```python
from build123d import *

# Parameters (mm, degrees)
SKETCH3_W               = 200
SKETCH3_H               = 160
BOSS_EXTRUDE1_DEPTH     = 4
SKETCH4_R               = 2
CUT_EXTRUDE1_DEPTH      = 129.124939024
CUT_EXTRUDE3_DEPTH      = 129.124939024
CUT_EXTRUDE3_DEPTH_BACK = 129.124939024
SKETCH5_W               = 30
SKETCH5_H               = 8
SKETCH7_W               = 25
SKETCH7_H               = 74
CUT_EXTRUDE4_DEPTH      = 129.124939024
CUT_EXTRUDE6_DEPTH      = 129.124939024
CUT_EXTRUDE6_DEPTH_BACK = 4
SKETCH12_W              = 8
SKETCH12_H              = 120
CUT_EXTRUDE8_DEPTH      = 129.124939024
SKETCH14_W              = 8
SKETCH14_H              = 120
CUT_EXTRUDE9_DEPTH      = 129.124939024
SKETCH15_W              = 8
SKETCH15_H              = 40
CUT_EXTRUDE10_DEPTH     = 129.124939024
SKETCH16_W              = 35
SKETCH16_H              = 8
CUT_EXTRUDE11_DEPTH     = 129.124939024


with BuildPart() as part:
    # Sketch3 → Boss-Extrude1 (new body)
    with BuildSketch(Plane(origin=(0, 0, 0), x_dir=(1, 0, 0), z_dir=(0, 1, 0))):
        Rectangle(SKETCH3_W, SKETCH3_H)
    extrude(amount=BOSS_EXTRUDE1_DEPTH)

    # Sketch4 → Cut-Extrude1 (cut, through all)
    with BuildSketch(Plane(origin=(0, 4, 0), x_dir=(1, 0, 0), z_dir=(0, 1, 0))):
        with Locations(Location((-93, 73, 0), (0, 0, 270))):
            Circle(SKETCH4_R)
        with Locations(Location((93, 73, 0), (0, 0, 270))):
            Circle(SKETCH4_R)
        with Locations(Location((-93, -73, 0), (0, 0, 270))):
            Circle(SKETCH4_R)
        with Locations(Location((93, -73, 0), (0, 0, 270))):
            Circle(SKETCH4_R)
    extrude(amount=-CUT_EXTRUDE1_DEPTH, mode=Mode.SUBTRACT)

    # Sketch5 → Cut-Extrude3 (cut, two sides: drawn at the far end of the back side and taken through both)
    with BuildSketch(Plane(origin=(0, 4, 0), x_dir=(1, 0, 0), z_dir=(0, 1, 0)).offset(-CUT_EXTRUDE3_DEPTH_BACK)):
        with Locations((-85, 46)):
            Rectangle(SKETCH5_W, SKETCH5_H)
    extrude(amount=CUT_EXTRUDE3_DEPTH + CUT_EXTRUDE3_DEPTH_BACK, mode=Mode.SUBTRACT)

    # Sketch7 → Cut-Extrude4 (cut, through all)
    with BuildSketch(Plane(origin=(0, 4, 0), x_dir=(1, 0, 0), z_dir=(0, 1, 0))):
        with Locations((-82.5, 0)):
            Rectangle(SKETCH7_W, SKETCH7_H)
    extrude(amount=-CUT_EXTRUDE4_DEPTH, mode=Mode.SUBTRACT)

    # Sketch11 → Cut-Extrude6 (cut, two sides: drawn at the far end of the back side and taken through both)
    with BuildSketch(Plane(origin=(0, 4, 0), x_dir=(1, 0, 0), z_dir=(0, 1, 0)).offset(-CUT_EXTRUDE6_DEPTH_BACK)):
        Polygon((-587.074417675, -42), (-100, -42), (-70, -42), (-70, -50), (-100, -50), (-587.074417675, -50), (-1561.223253025, -50), (-1561.223253025, -42), align=None)
    extrude(amount=CUT_EXTRUDE6_DEPTH + CUT_EXTRUDE6_DEPTH_BACK, mode=Mode.SUBTRACT)

    # Sketch12 → Cut-Extrude8 (cut, through all)
    with BuildSketch(Plane(origin=(0, 4, 0), x_dir=(1, 0, 0), z_dir=(0, 1, 0))):
        with Locations((91, 0)):
            Rectangle(SKETCH12_W, SKETCH12_H)
    extrude(amount=-CUT_EXTRUDE8_DEPTH, mode=Mode.SUBTRACT)

    # Sketch14 → Cut-Extrude9 (cut, through all)
    with BuildSketch(Plane(origin=(0, 4, 0), x_dir=(1, 0, 0), z_dir=(0, 1, 0))):
        with Locations((38, 0)):
            Rectangle(SKETCH14_W, SKETCH14_H)
    extrude(amount=-CUT_EXTRUDE9_DEPTH, mode=Mode.SUBTRACT)

    # Sketch15 → Cut-Extrude10 (cut, through all)
    with BuildSketch(Plane(origin=(0, 4, 0), x_dir=(1, 0, 0), z_dir=(0, 1, 0))):
        with Locations((-56, -40)):
            Rectangle(SKETCH15_W, SKETCH15_H)
    extrude(amount=-CUT_EXTRUDE10_DEPTH, mode=Mode.SUBTRACT)

    # Sketch16 → Cut-Extrude11 (cut, through all)
    with BuildSketch(Plane(origin=(0, 4, 0), x_dir=(1, 0, 0), z_dir=(0, 1, 0))):
        with Locations((64.5, -56)):
            Rectangle(SKETCH16_W, SKETCH16_H)
    extrude(amount=-CUT_EXTRUDE11_DEPTH, mode=Mode.SUBTRACT)


solid = part.part
```
Geometry check sheet. Reference: the model listing, model coordinates, mm. A direction names the side the tool comes from. Give positions to 0.01 mm unless a question says otherwise; leave off trailing zeros. Order: outer loops, then holes, each group sorted by start corner. A loop starts at its lowest first (then second) coordinate and runs counter-clockwise, first axis right, second up. Notation, with made-up numbers: (55.5, -18.75) - (72.5, -18.75) arc R18 ccw to (72.5, -14.75) - close; hole circle Ø11 at (-40, 88.5). An arc over 180 degrees is marked (long way). Answer in a Markdown table with one row per item. Add a question column.
Q1. Material ranges on probe 1 along X at (y, z) = (1.05, -73); probe 2 along X at (y, z) = (1.6, 33.5); probe 3 along X at (y, z) = (3.05, -3.5), recorded low to high. Write a range as from..to.
Q2. Mould release check, pull along X, two halves, no side actions. Record for faces 1 (the flat face through (-1, 4, -1)), 2 (the flat face through (-70, 2, -46)), 3 (the flat face through (-83, 2, 37)): pulls with the +X half, pulls with the -X half, needs draft (parallel to the pull), parting line crosses it, or undercut.
Q3. Gauge pin test, flat ends, axial feed: pin 1 (5 mm diameter, centred on x = 93, z = -73, fed in from -Y); pin 2 (3.5 mm diameter, centred on x = 93, z = 73, fed in from +Y). Record the tip position at first contact, or that the pin passes through.
Q4. Tool access check on faces 4 (the flat face through (-85, 2, 42)), 5 (the flat face through (42, 2, 1)), 6 (the flat face through (-1, 2, -80)). Record the directions out of +Z, -Z, +X, -X, +Y, -Y that give a thin tool (end or side, any length) a straight path to the whole face; none if there is none.
Q5. Cross-section at A-A, the plane z = 46. Enter the section's corners in (x, y).
Q6. Cross-section at C-C, the plane z = 11. Enter the section's corners in (x, y), then the cut area to 3 significant figures.
Q7. Cross-section at B-B, the plane y = 1.1. Count the separate pieces of the cut face and the enclosed holes in it, then the cut area to 3 significant figures.
Check values:
| question | item | result |
|---|---|---|
| 1 | probe 1 | x = -100..-95, -91..91, 95..100 |
| 1 | probe 2 | x = -100..-95, -70..-60, -52..34, 42..87, 95..100 |
| 1 | probe 3 | x = -100..-95, -70..34, 42..87, 95..100 |
| 2 | face 1 | needs draft |
| 2 | face 2 | pulls with the -X half |
| 2 | face 3 | undercut |
| 3 | pin 1 | stops at y = 0 |
| 3 | pin 2 | passes through |
| 4 | face 4 | -X, +Y, -Y |
| 4 | face 5 | +Y, -Y |
| 4 | face 6 | -Z, +X, -X, +Y, -Y |
| 5 | outline | (-70, 0) - (-60, 0) - (-60, 4) - (-70, 4) - close; (-52, 0) - (34, 0) - (34, 4) - (-52, 4) - close; (42, 0) - (87, 0) - (87, 4) - (42, 4) - close; (95, 0) - (100, 0) - (100, 4) - (95, 4) - close |
| 6 | outline | (-100, 0) - (-95, 0) - (-95, 4) - (-100, 4) - close; (-70, 0) - (34, 0) - (34, 4) - (-70, 4) - close; (42, 0) - (87, 0) - (87, 4) - (42, 4) - close; (95, 0) - (100, 0) - (100, 4) - (95, 4) - close |
| 6 | area | 636 mm^2 |
| 7 | separate pieces | 1 |
| 7 | enclosed holes | 9 |
| 7 | area | 27,100 mm^2 |
